Input: dimensioned drawing with shaded views. Units: mm. Origin: part minimum x, y, z. Coordinates: 2 decimals unless noted, no trailing zeros. Order: outer loops, then holes, each group sorted by start corner. A loop starts at its lowest first (then second) coordinate and runs counter-clockwise, first axis right, second up. Notation, with made-up numbers: M -15,27.5 L 6,27.5 A16 cw 6,44.5 Z; hole C -20.5,30 d4. An arc over 180 degrees is marked long. Write item = value, one per line.
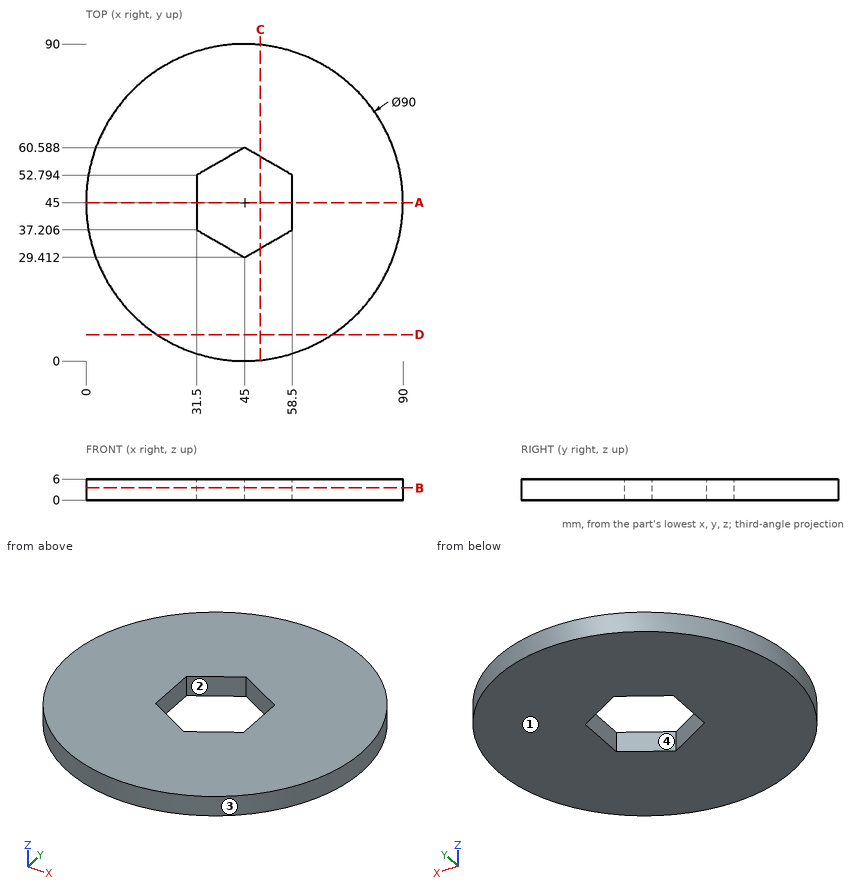
1) Section B-B, the plane z = 3.5. Return loops of the section in (x, y) (1 decimal), and give its area (3 significant figures).
Numbers:
outline = C 45,45 d90; hole M 31.5,37.2 L 45,29.4 L 58.5,37.2 L 58.5,52.8 L 45,60.6 L 31.5,52.8 Z
area = 5,730 mm²
2) Section A-A, the plane y = 45. Return loops of the section in (x, z).
Numbers:
outline = M 0,0 L 31.5,0 L 31.5,6 L 0,6 Z; M 58.5,0 L 90,0 L 90,6 L 58.5,6 Z
3) Section D-D, the plane y = 7.5. Return loops of the section in (x, z) (1 decimal).
Numbers:
outline = M 20.1,0 L 69.9,0 L 69.9,6 L 20.1,6 Z
4) Line query: L1, parallel to Y at x = 53.5, z = 5.7; L2, parallel to X at y = 35.5, z = 5.65 (1 decimal); L3, parallel to Y at x = 57, z = 5.2. Output: solid intervals per line, ascending.
Numbers:
L1 = 0.81 to 34.32, 55.68 to 89.19
L2 = 1 to 34.5, 55.5 to 89
L3 = 1.63 to 36.34, 53.66 to 88.37
5) Section C-C, the plane x = 49.5. Return loops of the section in (y, z) (1 decimal).
Numbers:
outline = M 0.2,0 L 32,0 L 32,6 L 0.2,6 Z; M 58,0 L 89.8,0 L 89.8,6 L 58,6 Z
6) Mould query, pull axis X, two halves, no side actions, for the marked faces 1, 2, 3 and 4. Classes: pulls with the +X half, pulls with the -X half, needs draft (parallel to the pull), parting line crosses it, or undercut.
Numbers:
face_1 = needs draft
face_2 = undercut
face_3 = parting line crosses it
face_4 = undercut
7) Pin query (flat end, axial travel): pin 1 (1 mm diameter, centred on x = 57, z = 2, fed in from -Y) (1 decimal); pin 2 (8 mm diameter, centred on x = 58.5, y = 61, fed in from -Z); pin 3 (2 mm diameter, centred on y = 38, z = 2, fed in from +X). Return the tip coordinate at first contact, or that it passes through.
Numbers:
pin_1 = 1.5
pin_2 = 0
pin_3 = 89.6
